Geometry: final body of the model. Coordinates: model frame, mm. A direction names the side the tool comes from. Round coordinates to 2 decimals unless told otherwise and drop trailing zeros. Write each loop counter-clockwise with the first axis right and the second up, starting at its lowest first coordinate (ties: lowest second). Pieces come first, ordered by that corner, then holes. Notation, with made-up numbers: M 40,23.5 L 50,23.5 A23 cw 50,31.5 Z; hole C 38.25,22.5 d8. An arc over 180 degrees is marked long. Use one line per item in the form item = value. Start each with the question number.
Item 1: Section query A-A (x = 0). Return loops of the section in (y, z).
Item 2: Pull-direction query (Y, two-part tool) for faces 3 (the cylindrical face through (2.872, 6.565, 2.465)), 4 (the flat face through (-45, 24, 2)), 5 (the flat face through (2, 50, 47)), 6 (the flat face through (1, 45, 49)); classes: pulls with the +Y half, pulls with the -Y half, needs draft (parallel to the pull), parting line crosses it, or undercut.
Item 3: Reachability of faces 1 (the flat face through (2, 3, 0)), 2 (the flat face through (45, -1, 49)) from +Z, -Z, +X, -X, +Y, -Y: full face, straight path, thin tool, end or side. Return the list, or none.
Item 4: Pin query (flat end, axial travel): pin 1 Ø6 at (x, y) = (26.5, -18) entering from +Z; pin 2 Ø10 at (x, z) = (-32.5, 20) entering from -Y; pin 3 Ø12 at (y, z) = (8, 77) entering from -X; pin 4 Ø10 at (x, y) = (-23, -9.5) entering from -Z. Return the tip coordinate at first contact, or that it passes through.
Item 5: Section query D-D (x = -22). Return loops of the section in (y, z), and give its area (3 significant figures).
Item 6: Ray query, probe 1 along Y at (x, z) = (0, 3.3); probe 2 along Z at (x, y) = (-5.5, -1.5); probe 3 along Y at (x, z) = (-29, 60). Return the intervals inside material, ascending.
Item 7: Section query B-B (y = 19.5). Return loops of the section in (x, z).
Item 8: Section query C-C (z = 62). Return loops of the section in (x, y).
from build123d import *

# Parameters (mm, degrees)
SKETCH1_W           = 100
SKETCH1_H           = 100
BOSS_EXTRUDE1_DEPTH = 5
BOSS_EXTRUDE2_DEPTH = 95
SKETCH3_R           = 13.25
CUT_EXTRUDE1_DEPTH  = 95
CUT_EXTRUDE2_DEPTH  = 123.474487139
SKETCH5_W           = 5
SKETCH5_H           = 95
CUT_EXTRUDE3_DEPTH  = 147.714007511


with BuildPart() as part:
    # Sketch1 → Boss-Extrude1 (new body)
    with BuildSketch(Plane.XY):
        Rectangle(SKETCH1_W, SKETCH1_H)
    extrude(amount=BOSS_EXTRUDE1_DEPTH)

    # Sketch2 → Boss-Extrude2 (add)
    with BuildSketch(Plane.XY.offset(5)):
        Polygon((-50, 50), (50, 50), (50, -50), (45, -50), (45, 45), (-50, 45), align=None)
    extrude(amount=BOSS_EXTRUDE2_DEPTH)

    # Sketch3 → Cut-Extrude1 (cut)
    with BuildSketch(Plane(origin=(0, 0, 0), x_dir=(-1, 0, 0), z_dir=(0, 0, -1))):
        with Locations((0, 19.5)):
            Circle(SKETCH3_R)
    extrude(amount=-CUT_EXTRUDE1_DEPTH, mode=Mode.SUBTRACT)

    # Sketch4 → Cut-Extrude2 (cut, through all)
    with BuildSketch(Plane(origin=(0, 0, 0), x_dir=(-1, 0, 0), z_dir=(0, 0, -1))):
        Polygon((-50, -50), (50, -50), (50, 50), (45, 50), (45, -45), (-50, -45), align=None)
    extrude(amount=-CUT_EXTRUDE2_DEPTH, mode=Mode.SUBTRACT)

    # Sketch5 → Cut-Extrude3 (cut, through all)
    with BuildSketch(Plane(origin=(50, 0, 0), x_dir=(0, 0, -1), z_dir=(1, 0, 0))):
        with Locations((-97.5, 2.5)):
            Rectangle(SKETCH5_W, SKETCH5_H)
    extrude(amount=-CUT_EXTRUDE3_DEPTH, mode=Mode.SUBTRACT)


solid = part.part
Working result:
q1.outline = M -45,0 L 6.25,0 L 6.25,5 L -45,5 Z; M 32.75,0 L 50,0 L 50,95 L 45,95 L 45,5 L 32.75,5 Z
q2.face_3 = undercut
q2.face_4 = needs draft
q2.face_5 = pulls with the +Y half
q2.face_6 = pulls with the -Y half
q3.face_1 = -Z, +X, -X, +Y, -Y
q3.face_2 = +Z, -X, -Y
q4.pin_1 = 5
q4.pin_2 = 45
q4.pin_3 = 45
q4.pin_4 = 0
q5.outline = M -45,0 L 50,0 L 50,95 L 45,95 L 45,5 L -45,5 Z
q5.area = 925 mm²
q6.probe_1 = -45 to 6.25, 32.75 to 50
q6.probe_2 = 0 to 5
q6.probe_3 = 45 to 50
q7.outline = M -45,0 L -13.25,0 L -13.25,5 L -45,5 Z; M 13.25,0 L 50,0 L 50,95 L 45,95 L 45,5 L 13.25,5 Z
q8.outline = M -45,45 L 45,45 L 45,-45 L 50,-45 L 50,50 L -45,50 Z
